Verification items for the finished model (mm, model axes). Face numbers are marked on the shaded views. A direction names the side the tool comes from. Coordinates: 2 decimals unless noted, no trailing zeros. Write each loop counter-clockwise with the first axis right and the second up, starting at its lowest first coordinate (ties: lowest second). Pieces come first, ordered by that corner, then holes. Notation, with made-up numbers: (83.5, -31.75) -> (136.5, -31.75) arc R17 ccw to (136.5, -14.75) -> close; hole circle Ø8 at (-34.5, 86). An arc over 180 degrees is marked (long way). Use a Markdown table: item, result. Add a question column.
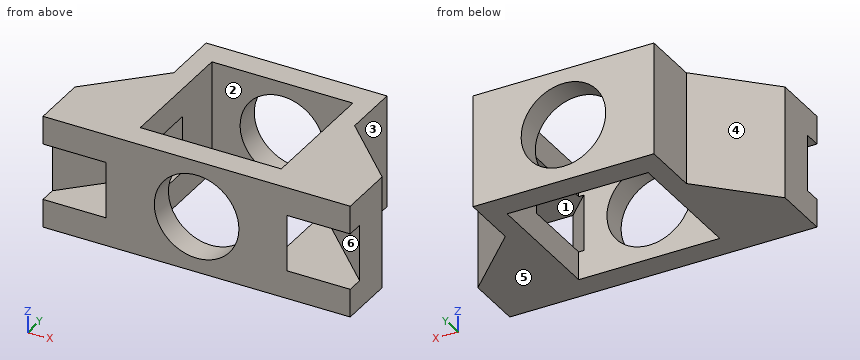
from build123d import *

# Parameters (mm, degrees)
SKETCH2_R           = 19.05
BOSS_EXTRUDE1_DEPTH = 152.4
BOSS_EXTRUDE2_DEPTH = 12.7
SKETCH4_W           = 138.346275672
SKETCH4_H           = 79.731841005
BOSS_EXTRUDE3_DEPTH = 50.8
SKETCH5_W           = 63.5
SKETCH5_H           = 57.15
CUT_EXTRUDE1_DEPTH  = 132.116075905
CUT_EXTRUDE2_DEPTH  = 132.116075905


with BuildPart() as part:
    # Sketch2 → Boss-Extrude1 (new body)
    with BuildSketch(Plane(origin=(0, 0, 0), x_dir=(1, 0, 0), z_dir=(0, 1, 0))):
        with Locations(Location((0, 0, 0), (0, 0, 90))):
            Circle(SKETCH2_R)
    extrude(amount=BOSS_EXTRUDE1_DEPTH)

    # Sketch3 → Boss-Extrude2 (add, symmetric)
    with BuildSketch(Plane.XY):
        Polygon((-427.750314484, -331.6732), (-409.789802242, -313.712687758), (-391.82929, -331.6732), align=None)
        Polygon((-6.028675512, 90.048438972), (-409.789802242, -313.712687758), (-391.82929, -331.6732), (11.93183673, 72.08792673), align=None)
    boss_extrude2 = extrude(amount=BOSS_EXTRUDE2_DEPTH, both=True)

    # Mirror1: Boss-Extrude2 across plane
    add(boss_extrude2.mirror(Plane(origin=(0, 0, 0), x_dir=(0, 0, 1), z_dir=(1, 0, 0))))


with BuildPart() as body_2:
    # Sketch4 → Boss-Extrude3 (new body)
    with BuildSketch(Plane.XY.offset(25.4)):
        with Locations((0, 59.259567455)):
            Rectangle(SKETCH4_W, SKETCH4_H)
    extrude(amount=-BOSS_EXTRUDE3_DEPTH)

    # Combine1: cut part
    add(part.part, mode=Mode.SUBTRACT)

    # Sketch5 → Cut-Extrude1 (cut, through all)
    with BuildSketch(Plane.XY.offset(25.4)):
        with Locations((0, 59.259567454)):
            Rectangle(SKETCH5_W, SKETCH5_H)
    extrude(amount=-CUT_EXTRUDE1_DEPTH, mode=Mode.SUBTRACT)

    # Sketch6 → Cut-Extrude2 (cut, through all)
    with BuildSketch(Plane.XY.offset(25.4)):
        Polygon((-69.173137836, 99.125487957), (-69.173137836, 44.864488891), (-40.730256121, 73.307370605), (-40.730256121, 99.125487957), align=None)
    cut_extrude2 = extrude(amount=-CUT_EXTRUDE2_DEPTH, mode=Mode.SUBTRACT)

    # Mirror2: Cut-Extrude2 across plane
    add(cut_extrude2.mirror(Plane(origin=(0, 0, 0), x_dir=(0, 0, 1), z_dir=(1, 0, 0))), mode=Mode.SUBTRACT)


solid = body_2.part
1) Cross-section at B-B on z = -22. Record the boundary of the cut face in (x, y), then the cut area to 3 significant figures.
2) Cross-section at D-D on z = 0. Record the boundary of the cut face in (x, y), then the cut area to 3 significant figures.
3) Release check for a two-part mould opening along Y. For the marked faces 4, 5 and 6 record: released by +Y, released by -Y, zero draft, split by the parting line, or undercut.
4) Cross-section at A-A on y = 84. Record the boundary of the cut face in (x, z), then the cut area to 3 significant figures.
5) Thickness scan on L1, parallel to X at y = 80, z = 21; L2, parallel to Y at x = -18, z = 21.5; L3, parallel to X at y = 28, z = 0. Record the ranges inside material, lowest first.
6) Gauge pin test, flat ends, axial feed: pin 1 (8 mm diameter, centred on y = 55, z = -4, fed in from +X); pin 2 (23 mm diameter, centred on x = 0, z = 0, fed in from +Y); pin 3 (1 mm diameter, centred on y = 82, z = 18, fed in from -X); pin 4 (15 mm diameter, centred on y = 62.5, z = 3, fed in from +X). Record the tip position at first contact, or that the pin passes through.
7) Cross-section at C-C on x = -27. Record the boundary of the cut face in (y, z), then the cut area to 3 significant figures.
8) Set-up check for the marked faces 1, 2 and 3: record each of +Z, -Z, +X, -X, +Y, -Y from which the full face is reachable in a straight line by a thin tool's end or side.
Returned:
| question | item | result |
|---|---|---|
| 1 | outline | (-69.17, 19.39) -> (69.17, 19.39) -> (69.17, 44.86) -> (40.73, 73.31) -> (40.73, 99.13) -> (-40.73, 99.13) -> (-40.73, 73.31) -> (-69.17, 44.86) -> close; hole (-31.75, 30.68) -> (31.75, 30.68) -> (31.75, 87.83) -> (-31.75, 87.83) -> close |
| 1 | area | 5,120 mm² |
| 2 | outline | (-69.17, 26.9) -> (-31.75, 64.33) -> (-31.75, 87.83) -> (-19.05, 87.83) -> (-19.05, 99.13) -> (-40.73, 99.13) -> (-40.73, 73.31) -> (-69.17, 44.86) -> close; (-40.76, 19.39) -> (-19.05, 19.39) -> (-19.05, 30.68) -> (-29.47, 30.68) -> close; (19.05, 19.39) -> (40.76, 19.39) -> (29.47, 30.68) -> (19.05, 30.68) -> close; (19.05, 87.83) -> (31.75, 87.83) -> (31.75, 64.33) -> (69.17, 26.9) -> (69.17, 44.86) -> (40.73, 73.31) -> (40.73, 99.13) -> (19.05, 99.13) -> close |
| 2 | area | 2,380 mm² |
| 3 | face 4 | released by +Y |
| 3 | face 5 | zero draft |
| 3 | face 6 | undercut |
| 4 | outline | (-40.73, -25.4) -> (-31.75, -25.4) -> (-31.75, 25.4) -> (-40.73, 25.4) -> close; (31.75, -25.4) -> (40.73, -25.4) -> (40.73, 25.4) -> (31.75, 25.4) -> close |
| 4 | area | 912 mm² |
| 5 | L1 | x = -40.73 to -31.75, 31.75 to 40.73 |
| 5 | L2 | y = 19.39 to 30.68, 87.83 to 99.13 |
| 5 | L3 | x = -69.17 to -68.08, -32.16 to -19.05, 19.05 to 32.16, 68.08 to 69.17 |
| 6 | pin 1 | stops at x = 63.04 |
| 6 | pin 2 | passes through |
| 6 | pin 3 | stops at x = -40.73 |
| 6 | pin 4 | stops at x = 59.04 |
| 7 | outline | (19.39, -25.4) -> (30.68, -25.4) -> (30.68, 25.4) -> (19.39, 25.4) -> close; (87.83, -25.4) -> (99.13, -25.4) -> (99.13, 25.4) -> (87.83, 25.4) -> close |
| 7 | area | 1,150 mm² |
| 8 | face 1 | none |
| 8 | face 2 | +Z, -Z |
| 8 | face 3 | +Z, -Z, +X, +Y |
